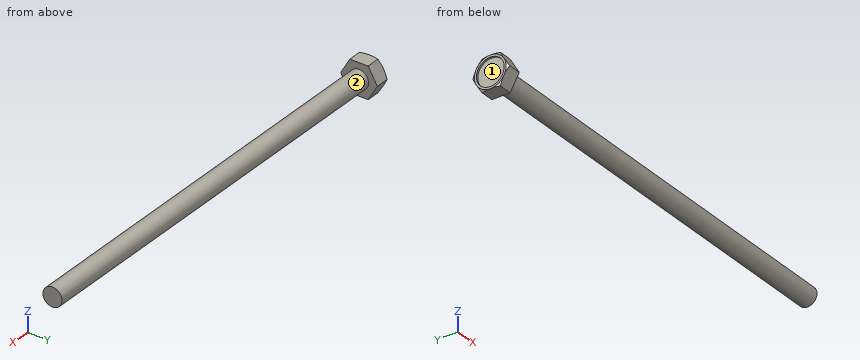
```python
from build123d import *

# Parameters (mm, degrees)
SKETCH2_R     = 2.915704388
HEX_DIE_DEPTH = 2.3
SKETCH4_R     = 2.1875
INDENT_DEPTH  = 0.2875


with BuildPart() as part:
    # BodySke → Base-Revolve (revolve)
    with BuildSketch(Plane.XY):
        Polygon((2.3, 1.5), (2.3, 2.886836028), (0.223339885, 2.886836028), (0, 2.5), (0, 0), (68.3, 0), (68.3, 1.5), align=None)
    revolve(axis=Axis((-25.4, 0, 0), (1, 0, 0)))

    # Sketch2 → Hex-Die (cut)
    with BuildSketch(Plane(origin=(0, 0, 0), x_dir=(0, 0, -1), z_dir=(1, 0, 0))):
        Circle(SKETCH2_R)
        Polygon((-2.5, 1.443375679), (0, 2.886751359), (2.5, 1.443375679), (2.5, -1.443375679), (0, -2.886751359), (-2.5, -1.443375679), align=None, mode=Mode.SUBTRACT)
    extrude(amount=HEX_DIE_DEPTH, mode=Mode.SUBTRACT)

    # Sketch4 → Indent (cut)
    with BuildSketch(Plane(origin=(0, 0, 0), x_dir=(0, 0, -1), z_dir=(1, 0, 0))):
        Circle(SKETCH4_R)
    extrude(amount=INDENT_DEPTH, mode=Mode.SUBTRACT)


solid = part.part
```
Build history of the part. All positions in model axes, mm. Face numbers are marked on the shaded views. Coordinates: 2 decimals unless noted, no trailing zeros. Write each loop counter-clockwise with the first axis right and the second up, starting at its lowest first coordinate (ties: lowest second). Pieces come first, ordered by that corner, then holes.
1. Drill centre lines: probe 1 along X at (y, z) = (-1.45, -1.1); probe 2 along X at (y, z) = (1.2, 0.3); probe 3 along Y at (x, z) = (51, 0.85). Where is each one in solid material? Low to high.
Answer block:
probe 1: x = 0.29 to 2.3
probe 2: x = 0.29 to 68.3
probe 3: y = -1.24 to 1.24
2. Pull direction Z, two halves, no side cores. Call the marked faces 1 and 2: released by +Z, released by -Z, zero draft, split by the parting line, or undercut.
Answer block:
face 1: undercut
face 2: split by the parting line
3. Drop flat-ended pins along their axis: pin 1 (1 mm diameter, centred on x = 28, z = -1, fed in from -Y); pin 2 (1.5 mm diameter, centred on x = 20, z = 2, fed in from +Y); pin 3 (3 mm diameter, centred on x = 9.5, y = -0.5, fed in from -Z). Give the stop position or say it passes through.
Answer block:
pin 1: stops at y = -1.41
pin 2: stops at y = 0.83
pin 3: stops at z = -1.5
4. Band-saw the part on A-A, the plane x = 53. Give the cut face in (y, z).
Answer block:
outline: circle Ø3 at (0, 0)
